Autodesk Inventor part; units mm, degrees
ref_plane "YZ Plane" through (0, 0, 0) normal (1, 0, 0) x (0, 1, 0)
ref_plane "XZ Plane" through (0, 0, 0) normal (0, 1, 0) x (-1, 0, 0)
ref_plane "XY Plane" through (0, 0, 0) normal (0, 0, 1) x (1, 0, 0)
sketch "Sketch1" plane through (0, 0, 0) normal (0, 1, 0) x (-1, 0, 0)
  circle A0 centre (0, 0) radius 1.5875
  dimension "d0" = 3.175
extrude "Extrusion1" add sketch "Sketch1" along normal blind 254
sketch "Sketch2" plane through (0, 254, 0) normal (0, 1, 0) x (1, 0, 0)
  circle A0 centre (0, 0) radius 1.5875
hole "Hole1" at (0, 254, 0) direction (0, -1, 0) diameter 2.159 end through all
sketch "Sketch3" plane through (0, 0, 0) normal (0, 0, 1) x (1, 0, 0)
  line L0 (1.5875, 0) -> (-1.5875, 0)
  line L1 (0, 0) -> (0, 6.35)
  line L2 (0, 0) -> (6.35, 0) construction
  line L3 (0, 6.35) -> (0, 8.89)
  line L4 (0, 8.89) -> (0, 12.7)
  line L5 (0, 8.89) -> (3.81, 8.89) construction
  circle A0 centre (0, 12.7) radius 0.635
  dimension "d10" = 6.35
  dimension "d11" = 270
  dimension "d12" = 2.54
  dimension "d13" = 3.81
  dimension "d14" = 90
  dimension "d15" = 1.27
sketch "Sketch4" plane through (0, 0, 0) normal (0, 1, 0) x (-1, 0, 0)
  point P0 (0, 0)
sketch "Sketch5" plane through (0, 0, 0) normal (0, 0, 1) x (1, 0, 0)
  line L0 (-1.0795, 254) -> (1.0795, 254)
  line L1 (0, 254) -> (0, 241.3)
  circle A0 centre (0, 241.3) radius 0.635
  point P0 (0, 0)
  dimension "d16" = 12.7
  dimension "d17" = 1.27
hole "Hole2" at (0, 241.3, 0) direction (0, 0, -1) diameter 1.27 depth 1.5875 tip angle 118
hole "Hole3" at (0, 12.7, 0) direction (0, 0, -1) diameter 1.27 depth 1.5875 tip angle 118
sketch "Sketch6" plane through (0, 0, 0) normal (1, 0, 0) x (0, 1, 0)
  point P0 (0, 0)
properties part number "burder_rod_2"
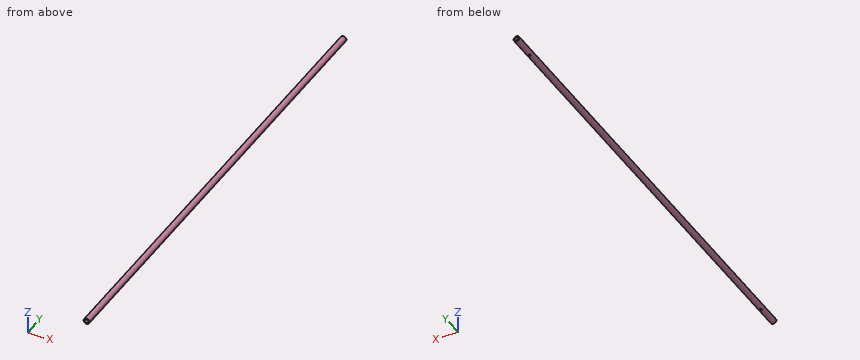
Can you work these out from the model? Positions are in its coordinate system, mm. Round coordinates to 2 decimals unless told otherwise and drop trailing zeros. Order: outer loops, then holes, each group sorted by start corner. A loop starts at its lowest first (then second) coordinate and runs counter-clockwise, first axis right, second up. Notation, with made-up numbers: (21.5, 39) -> (61.5, 39) arc R31 cw to (61.5, 71) -> close; hole circle Ø4 at (74, 24.25). An arc over 180 degrees is marked (long way). Return JSON: item names as keys, results as strings. Group by question number.
1. Will this pin go through, and if not, where does the flat tip stop? pin 1 (1.3 mm diameter, centred on x = 0, z = 0, fed in from -Y).
2. I need wall thicknesses on line 1 (Y direction, x = 0, z = -1.4) (3 decimals); line 2 (Z direction, x = 0.15, y = 25). Which ranges of each line are inside material? Lowest first, please. Write a range as [from, to].
3. If we section it at B-B, the plane x = 0: Write out the boundary of the cut face in (y, z) (1 decimal), then the cut area to 3 significant figures.
4. If we section it at A-A, the plane z = 0: Write out the boundary of the cut face in (x, y), then the cut area to 3 significant figures.
5. If we section it at C-C, the plane y = 62: Write out the boundary of the cut face in (x, z) (1 decimal), then the cut area to 3 significant figures.
Output values:
{
 "1": {"pin 1": "through"},
 "2": {"line 1": "[0, 12.065], [13.335, 240.665], [241.935, 254]", "line 2": "[-1.58, -1.07], [1.07, 1.58]"},
 "3": {"outline": "(0, -1.6) -> (12.1, -1.6) -> (12.1, -1.1) -> (0, -1.1) -> close; (0, 1.1) -> (254, 1.1) -> (254, 1.6) -> (0, 1.6) -> close; (13.3, -1.6) -> (240.7, -1.6) -> (240.7, -1.1) -> (13.3, -1.1) -> close; (241.9, -1.6) -> (254, -1.6) -> (254, -1.1) -> (241.9, -1.1) -> close", "area": "257 mm²"},
 "4": {"outline": "(-1.59, 0) -> (-1.08, 0) -> (-1.08, 254) -> (-1.59, 254) -> close; (1.08, 0) -> (1.59, 0) -> (1.59, 254) -> (1.08, 254) -> close", "area": "258 mm²"},
 "5": {"outline": "circle Ø3.2 at (0, 0); hole circle Ø2.2 at (0, 0)", "area": "4.26 mm²"}
}
